Could you check a few things on this model? Use its own coordinates, in mm. Give positions to 0.01 mm unless a question says otherwise; leave off trailing zeros. Order: outer loops, then holes, each group sorted by start corner. A loop starts at its lowest first (then second) coordinate and runs counter-clockwise, first axis right, second up.
(1) If we mould it in two halves opening along Y, with no side actions, what happens to faces 1 (the conical face through (79.756, -46.467, -209.254)), 2 (the flat face through (161.236, -4, 4)), 3 (the flat face through (98.847, -3, 3))? For each: released by +Y, released by -Y, zero draft, split by the parting line, or undercut.
(2) If I drill on probe 1 along X at (y, z) = (29, -49.5); probe 2 along Z at (x, y) = (140, 232.5); probe 3 along Z at (x, y) = (131.5, 144), over which ranges is the centre line in solid material (lowest first)?
(3) Will these pins go through, and if not, where does the flat tip stop? pin 1 (4 mm diameter, centred on x = 130.5, z = -89.5, fed in from -Y); pin 2 (1 mm diameter, centred on y = 118, z = 222, fed in from -X); pin 3 (1 mm diameter, centred on y = 39.5, z = -244, fed in from -X).
(4) Imagine slicing it at A-A, the plane x = 127. Write out the boundary of the cut face in (y, z), then the cut area to 3 significant figures.
Autodesk Inventor part; units mm, degrees
ref_plane "Work Plane1" through (0, 0, -10) normal (-1, 0, 0) x (0, -1, 0)
ref_plane "YZ Plane" through (0, 0, 0) normal (1, 0, 0) x (0, 1, 0)
ref_plane "XZ Plane" through (0, 0, 0) normal (0, 1, 0) x (-1, 0, 0)
ref_plane "Work Plane1" through (0, 0, -10) normal (-1, 0, 0) x (0, -1, 0)
sketch "Sketch1" plane through (0, 0, 0) normal (0, 0, 1) x (1, 0, 0)
  line L0 (-21.83974, 0) -> (131.038441, 0)
  line L1 (0, 0) -> (11.555806, 28.889516) construction
  line L2 (93.359081, 201.02678) -> (142.712708, 307.298186)
  line L3 (93.359081, 201.02678) -> (98.847306, 198.83149)
  line L4 (98.847306, 198.83149) -> (98.847306, 0)
  line L5 (142.712708, 307.298186) -> (161.235818, 299.888942)
  line L6 (161.235818, 299.888942) -> (161.235818, 0)
  dimension "delta" = 68.1986
  dimension "hxe" = 19.95
  dimension "hxi" = 5.911
  dimension "hfe" = 18.37774
  dimension "hfi" = 12.02226
  dimension "Ri" = 221.32137
  dimension "b" = 117
sketch "Sketch1 outline for Revolution1" plane through (0, 0, 0) normal (0, 0, 1) x (1, 0, 0)
  line L0 (98.847306, 198.83149) -> (98.847306, 0)
  line L1 (93.359081, 201.02678) -> (98.847306, 198.83149)
  line L2 (142.712708, 307.298186) -> (93.359081, 201.02678)
  line L3 (161.235818, 299.888942) -> (142.712708, 307.298186)
  line L4 (161.235818, 0) -> (161.235818, 299.888942)
  line L5 (98.847306, 0) -> (161.235818, 0)
revolve "Revolution1" add sketch "Sketch1 outline for Revolution1" angle 360 about axis through (-10, 0, 0) along (1, 0, 0)
sketch "Sketch2" plane through (0, 0, 0) normal (0, 0, 1) x (1, 0, 0)
  line L0 (-20.687045, 0) -> (124.12227, 0)
  line L1 (0, 0) -> (11.984241, 29.960604) construction
  line L2 (93.359081, 201.02678) -> (142.712708, 307.298186)
  line L3 (93.359081, 201.02678) -> (77.202995, 207.489214)
  line L4 (142.712708, 307.298186) -> (118.015819, 317.176941)
  line L5 (118.015819, 317.176941) -> (77.202995, 207.489214)
  dimension "hae" = 8.22162
  dimension "hai" = 5.37838
  dimension "d10" = 68.1986
revolve "Revolution2" add sketch "Sketch2" angle 360 about axis through (-10, 0, 0) along (1, 0, 0)
equation "\"delta\" = MC_delta2"
equation "\"hxe\" = MC_hxe2 + MC_hae2 - MC_h2E"
equation "\"hxi\" = MC_hxi2 + MC_hai2 - MC_h2A"
equation "\"hfe\" = MC_h2E - MC_hae2"
equation "\"hfi\" = MC_h2A - MC_hai2"
equation "\"Ri\" = MC_Ri"
equation "\"b\" = MC_b"
equation "\"hae\" = MC_hae2"
equation "\"hai\" = MC_hai2"
equation "\"d10\" = delta"
equation "\"SumDelta\" = MC_deltasum"
equation "\"MC_deltasum\" = 90deg"
equation "\"MC_b\" = 117"
equation "\"MC_Ri\" = 221.32137"
equation "\"MC_alfa\" = 20deg"
equation "\"MC_delta1\" = 21.801409deg"
equation "\"MC_hae1\" = 15.95962"
equation "\"MC_hxe1\" = 23.93975"
equation "\"MC_hai1\" = 10.44038"
equation "\"MC_hxi1\" = 11.79625"
equation "\"MC_delta2\" = 68.1986deg"
equation "\"MC_hae2\" = 8.22162"
equation "\"MC_hxe2\" = 38.32774"
equation "\"MC_hai2\" = 5.37838"
equation "\"MC_hxi2\" = 17.93326"
equation "\"MC_Ang1A\" = 203.543093deg"
equation "\"MC_Ang1B\" = 190.397416deg"
equation "\"MC_Ang1C\" = 180deg"
equation "\"MC_Ang1D\" = 171.570572deg"
equation "\"MC_Ang1E\" = 164.598698deg"
equation "\"MC_Ang2A\" = 170.582763deg"
equation "\"MC_Ang2B\" = 175.841034deg"
equation "\"MC_Ang2C\" = 180deg"
equation "\"MC_Ang2D\" = 183.371771deg"
equation "\"MC_Ang2E\" = 186.160521deg"
equation "\"MC_h1A\" = 17.40064"
equation "\"MC_h1B\" = 19.70032"
equation "\"MC_h1C\" = 22"
equation "\"MC_h1D\" = 24.29968"
equation "\"MC_h1E\" = 26.59936"
equation "\"MC_h2A\" = 17.40064"
equation "\"MC_h2B\" = 19.70032"
equation "\"MC_h2C\" = 22"
equation "\"MC_h2D\" = 24.29968"
equation "\"MC_h2E\" = 26.59936"
equation "\"MC_Rz1A\" = 82.19669"
equation "\"MC_Rz1B\" = 93.05987"
equation "\"MC_Rz1C\" = 103.92305"
equation "\"MC_Rz1D\" = 114.78623"
equation "\"MC_Rz1E\" = 125.6494"
equation "\"MC_Rz2A\" = 205.49173"
equation "\"MC_Rz2B\" = 232.64968"
equation "\"MC_Rz2C\" = 259.80762"
equation "\"MC_Rz2D\" = 286.96556"
equation "\"MC_Rz2E\" = 314.12351"
equation "\"MC_Sa1A\" = 2.90562"
equation "\"MC_Sa1B\" = 3.28962"
equation "\"MC_Sa1C\" = 3.67363"
equation "\"MC_Sa1D\" = 4.05764"
equation "\"MC_Sa1E\" = 4.44165"
equation "\"MC_Sa2A\" = 4.42236"
equation "\"MC_Sa2B\" = 5.00682"
equation "\"MC_Sa2C\" = 5.59128"
equation "\"MC_Sa2D\" = 6.17574"
equation "\"MC_Sa2E\" = 6.7602"
equation "\"MC_tx1A\" = 13.29713"
equation "\"MC_tx1B\" = 15.05449"
equation "\"MC_tx1C\" = 16.81185"
equation "\"MC_tx1D\" = 18.56921"
equation "\"MC_tx1E\" = 20.32657"
equation "\"MC_tx2A\" = 10.0867"
equation "\"MC_tx2B\" = 11.41977"
equation "\"MC_tx2C\" = 12.75284"
equation "\"MC_tx2D\" = 14.0859"
equation "\"MC_tx2E\" = 15.41897"
equation "\"MC_bD\" = 29.25"
equation "\"MC_bC\" = 58.5"
equation "\"MC_bB\" = 87.75"
equation "\"MC_bA\" = 119.34"
equation "\"MC_mx1A\" = 7.47431"
equation "\"MC_mx1B\" = 8.46212"
equation "\"MC_mx1C\" = 9.44993"
equation "\"MC_mx1D\" = 10.43775"
equation "\"MC_mx1E\" = 11.42556"
equation "\"MC_mx2A\" = 7.05073"
equation "\"MC_mx2B\" = 7.98256"
equation "\"MC_mx2C\" = 8.91439"
equation "\"MC_mx2D\" = 9.84622"
equation "\"MC_mx2E\" = 10.77805"
properties part number "bevelgear_wheel2"
Answer block:
1. face 1: split by the parting line
1. face 2: zero draft
1. face 3: undercut
2. probe 1: x = 98.85 to 161.24
2. probe 2: z = -202.59 to 202.59
2. probe 3: z = -276.54 to 276.54
3. pin 1: stops at y = -300.1
3. pin 2: stops at x = 93.36
3. pin 3: stops at x = 91.78
4. outline: circle Ø627.17 at (0, 0)
4. area: 309,000 mm2
